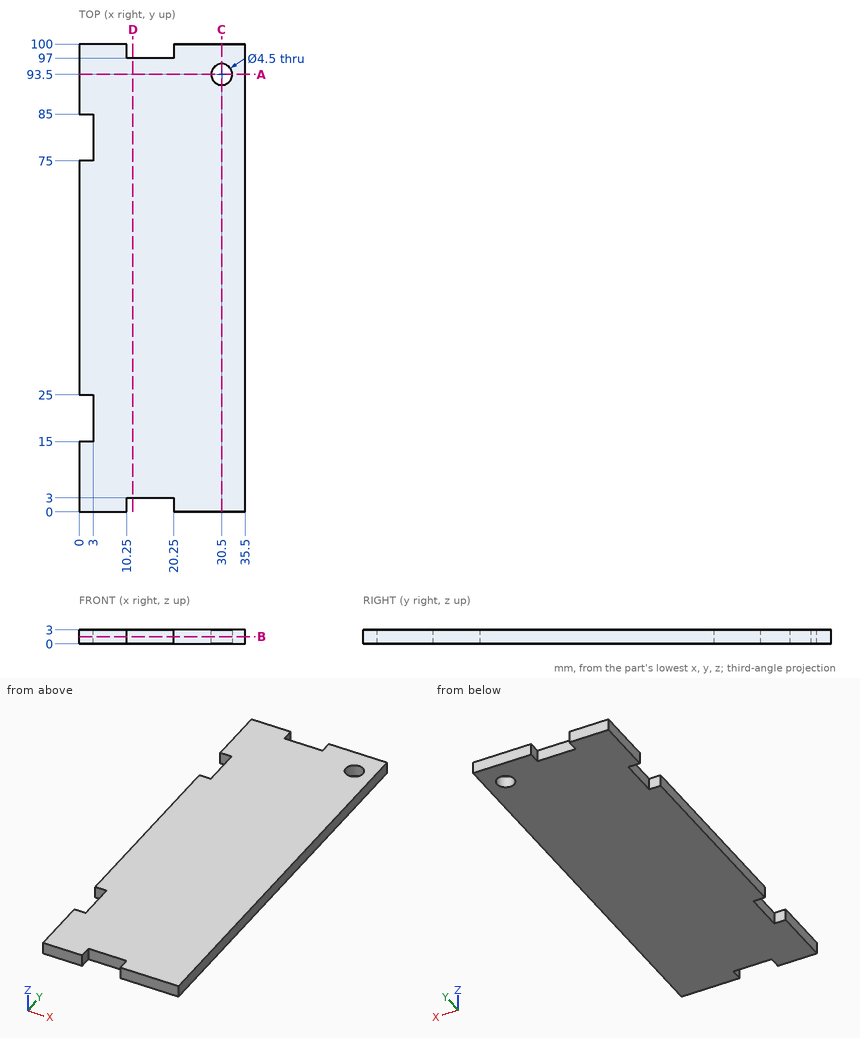
Design review of the part shown in the three views and the two pictorial views. Dimensions are in mm from the part's minimum x, y and z. Coordinates: 2 decimals unless noted, no trailing zeros. Order: outer loops, then holes, each group sorted by start corner. A loop starts at its lowest first (then second) coordinate and runs counter-clockwise, first axis right, second up. Notation, with made-up numbers: (-7, 29.5) -> (3, 29.5) arc R21 ccw to (3, 43.5) -> close; hole circle Ø4 at (-27.5, -35.75). An arc over 180 degrees is marked (long way). Use one line per item in the form item = value. Start each with the question number.
(1) Insertion check: pin 1 (0.9 mm diameter, centred on x = 15, z = 1.5, fed in from +Y); pin 2 (1.5 mm diameter, centred on y = 79, z = 1.5, fed in from -X). Each pin has a flat end and moves straight along its axis. Give the tip position at first contact, or say it passes through.
(2) Add section A-A on y = 93.5. State the section outline as (x, z) points.
(3) Add section C-C on x = 30.5. State the section outline as (y, z) points.
(4) Add section B-B on z = 1.55. State the section outline as (x, y) points.
(5) Add section D-D on x = 11.5. State the section outline as (y, z) points, plus the area to 3 significant figures.
(6) For probe 1 along X at (y, z) = (93.5, 1.9); probe 2 along Y at (x, z) = (30.5, 1.05); probe 3 along X at (y, z) = (78, 1), list the stretches that pass through material, from the lowest coordinate up.
Answer block:
q1.pin_1 = 97
q1.pin_2 = 3
q2.outline = (0, 0) -> (28.25, 0) -> (28.25, 3) -> (0, 3) -> close; (32.75, 0) -> (35.5, 0) -> (35.5, 3) -> (32.75, 3) -> close
q3.outline = (0, 0) -> (91.25, 0) -> (91.25, 3) -> (0, 3) -> close; (95.75, 0) -> (100, 0) -> (100, 3) -> (95.75, 3) -> close
q4.outline = (0, 0) -> (10.25, 0) -> (10.25, 3) -> (20.25, 3) -> (20.25, 0) -> (35.5, 0) -> (35.5, 100) -> (20.25, 100) -> (20.25, 97) -> (10.25, 97) -> (10.25, 100) -> (0, 100) -> (0, 85) -> (3, 85) -> (3, 75) -> (0, 75) -> (0, 25) -> (3, 25) -> (3, 15) -> (0, 15) -> close; hole circle Ø4.5 at (30.5, 93.5)
q5.outline = (3, 0) -> (97, 0) -> (97, 3) -> (3, 3) -> close
q5.area = 282 mm²
q6.probe_1 = 0 to 28.25, 32.75 to 35.5
q6.probe_2 = 0 to 91.25, 95.75 to 100
q6.probe_3 = 3 to 35.5
